```python
from build123d import *

# Parameters (mm, degrees)
SKETCH1_R           = 2.7
BOSS_EXTRUDE1_DEPTH = 9.23
SKETCH2_R           = 3.6
BOSS_EXTRUDE2_DEPTH = 0.5
SKETCH3_R           = 2.7
BOSS_EXTRUDE3_DEPTH = 1
BOSS_EXTRUDE4_DEPTH = 8.9


with BuildPart() as part:
    # Sketch1 → Boss-Extrude1 (new, symmetric)
    with BuildSketch(Plane.XY):
        Circle(SKETCH1_R)
    extrude(amount=BOSS_EXTRUDE1_DEPTH, both=True)

    # Sketch2 → Boss-Extrude2 (add)
    with BuildSketch(Plane.XY.offset(9.23)):
        Circle(SKETCH2_R)
    boss_extrude2 = extrude(amount=BOSS_EXTRUDE2_DEPTH)

    # Sketch3 → Boss-Extrude3 (add)
    with BuildSketch(Plane.XY.offset(9.73)):
        Circle(SKETCH3_R)
    boss_extrude3 = extrude(amount=BOSS_EXTRUDE3_DEPTH)

    # Sketch3_3 → Boss-Extrude4 (add)
    with BuildSketch(Plane.XY.offset(9.73)):
        with BuildLine():
            ThreePointArc((-2.01, 1.802747903), (-2.521606631, 0.965142477), (-2.7, 0))
            Line((-2.7, 0), (2.7, 0))
            ThreePointArc((2.7, 0), (2.521606631, 0.965142477), (2.01, 1.802747903))
            Line((2.01, 1.802747903), (-2.01, 1.802747903))
        make_face()
        with BuildLine():
            Line((2.7, 0), (-2.7, 0))
            ThreePointArc((-2.7, 0), (-2.521606631, -0.965142477), (-2.01, -1.802747903))
            Line((-2.01, -1.802747903), (2.01, -1.802747903))
            ThreePointArc((2.01, -1.802747903), (2.521606631, -0.965142477), (2.7, 0))
        make_face()
    boss_extrude4 = extrude(amount=BOSS_EXTRUDE4_DEPTH)

    # Mirror1: Boss-Extrude2, Boss-Extrude3, Boss-Extrude4 across plane
    add(boss_extrude2.mirror(Plane.XY))
    add(boss_extrude3.mirror(Plane.XY))
    add(boss_extrude4.mirror(Plane.XY))


solid = part.part
```
Model file for the job. Use its own axes, mm. A direction names the side the tool comes from. Give positions to 0.01 mm unless a question says otherwise; leave off trailing zeros. Loops run counter-clockwise (first coordinate to the right, second up) from the corner with the lowest first, then second, coordinate; pieces in that order, holes last. Notation, with made-up numbers: (46, -37.5) -> (60, -37.5) arc R23 ccw to (60, -29.5) -> close; hole circle Ø10 at (38.5, 70.5). An arc over 180 degrees is marked (long way). Write each question's results on one line, items separated by ' | '.
(1) Probe line 1 along Z through (x, y) = (-1.25, 2.5); line 2 along Z through (x, y) = (-0.25, -2); line 3 along X through (y, z) = (0, -17). List the from-to ranges inside material, lowest first.
Geometry results:
line 1: z = -9.73 to -9.23, 9.23 to 9.73 | line 2: z = -10.73 to 10.73 | line 3: x = -2.7 to 2.7
(2) Tool access for faces 4 (the flat face through (0, -2, -10.73)), 5 (the flat face through (1, 3, 9.73)), 6 (the flat face through (0, 2, 10.73)), 7 (the cylindrical face through (2.497, -1.028, -14.118)), 8 (the flat face through (1, 3, 9.23)): list every direction of +Z, -Z, +X, -X, +Y, -Y with a clear straight run to the whole face (end or side of a thin tool).
Geometry results:
face 4: -Z, +X, -X, -Y | face 5: +Z | face 6: +Z, +X, -X, +Y | face 7: -Z | face 8: none
(3) Pull direction Z, two halves, no side cores. Call faces 1 (the flat face through (0, 0, -18.63)), 2 (the cylindrical face through (-0.585, -2.636, 0.129)), 3 (the flat face through (0, -2, 10.73)): released by +Z, released by -Z, zero draft, split by the parting line, or undercut.
Geometry results:
face 1: released by -Z | face 2: undercut | face 3: released by +Z
(4) Flat gauge pins, fed straight in: pin 1 Ø3 at (x, z) = (-1, 15.5) entering from -Y; pin 2 Ø1 at (x, y) = (1, 2) entering from +Z; pin 3 Ø3 at (y, z) = (0.5, -3.5) entering from +X; pin 4 Ø1.5 at (x, z) = (-0.5, 14) entering from +Y. Where does each tip first touch, or does it go through?
Geometry results:
pin 1: stops at y = -1.8 | pin 2: stops at z = 18.63 | pin 3: stops at x = 2.7 | pin 4: stops at y = 1.8
(5) Cut at A-A on x = 0. List the corners of the cut face in (y, z), and give its area (3 significant figures).
Geometry results:
outline: (-3.6, -9.73) -> (-2.7, -9.73) -> (-2.7, -10.73) -> (-1.8, -10.73) -> (-1.8, -18.63) -> (1.8, -18.63) -> (1.8, -10.73) -> (2.7, -10.73) -> (2.7, -9.73) -> (3.6, -9.73) -> (3.6, -9.23) -> (2.7, -9.23) -> (2.7, 9.23) -> (3.6, 9.23) -> (3.6, 9.73) -> (2.7, 9.73) -> (2.7, 10.73) -> (1.8, 10.73) -> (1.8, 18.63) -> (-1.8, 18.63) -> (-1.8, 10.73) -> (-2.7, 10.73) -> (-2.7, 9.73) -> (-3.6, 9.73) -> (-3.6, 9.23) -> (-2.7, 9.23) -> (-2.7, -9.23) -> (-3.6, -9.23) -> close | area: 175 mm²
(6) Cut at B-B on z = -7. List the corners of the cut face in (x, y).
Geometry results:
outline: circle Ø5.4 at (0, 0)
